```python
from build123d import *

# Parameters (mm, degrees)
SKETCH1_R           = 15
SKETCH1_R_2         = 40
BOSS_EXTRUDE4_DEPTH = 51


with BuildPart() as part:
    # Sketch1 → Boss-Extrude4 (new body)
    # profile 1 of 3: a face of its own
    with BuildSketch(Plane.XY):
        with BuildLine():
            ThreePointArc((-29.002885891, 59.651863383), (-46.6282273, 80.727545655), (-70.02485881, 66.324952937))
            Line((-70.02485881, 66.324952937), (-89.071294105, 6.023764702))
            ThreePointArc((-89.071294105, 6.023764702), (-66.95253237, 19.766460003), (-50, 0))
            ThreePointArc((-50, 0), (-66.95253237, -19.766460003), (-89.071294105, -6.023764702))
            Line((-89.071294105, -6.023764702), (-70.02485881, -66.324952937))
            ThreePointArc((-70.02485881, -66.324952937), (-46.6282273, -80.727545655), (-29.002885891, -59.651863383))
            ThreePointArc((-29.002885891, -59.651863383), (-22.168588856, -44.262528341), (-6.003756239, -39.546869801))
            ThreePointArc((-6.003756239, -39.546869801), (-40, 0), (-6.003756239, 39.546869801))
            ThreePointArc((-6.003756239, 39.546869801), (-22.168588856, 44.262528341), (-29.002885891, 59.651863383))
        make_face()
        with Locations((-50, -60)):
            Circle(SKETCH1_R, mode=Mode.SUBTRACT)
        with Locations((-50, 60)):
            Circle(SKETCH1_R, mode=Mode.SUBTRACT)
    # profile 2 of 3: a face of its own
    with BuildSketch(Plane.XY):
        with BuildLine():
            ThreePointArc((29.002885891, 59.651863383), (22.168588856, 44.262528341), (6.003756239, 39.546869801))
            ThreePointArc((6.003756239, 39.546869801), (30.332740146, 26.075369129), (40, 0))
            ThreePointArc((40, 0), (30.332740146, -26.075369129), (6.003756239, -39.546869801))
            ThreePointArc((6.003756239, -39.546869801), (22.168588856, -44.262528341), (29.002885891, -59.651863383))
            ThreePointArc((29.002885891, -59.651863383), (46.6282273, -80.727545655), (70.02485881, -66.324952937))
            Line((70.02485881, -66.324952937), (89.071294105, -6.023764702))
            ThreePointArc((89.071294105, -6.023764702), (50, 0), (89.071294105, 6.023764702))
            Line((89.071294105, 6.023764702), (70.02485881, 66.324952937))
            ThreePointArc((70.02485881, 66.324952937), (46.6282273, 80.727545655), (29.002885891, 59.651863383))
        make_face()
        with Locations((50, -60)):
            Circle(SKETCH1_R, mode=Mode.SUBTRACT)
        with Locations((50, 60)):
            Circle(SKETCH1_R, mode=Mode.SUBTRACT)
    # profile 3 of 3: a face of its own
    with BuildSketch(Plane.XY):
        Circle(SKETCH1_R_2)
        with BuildLine():
            ThreePointArc((26.090759323, 18.527608533), (16, 27.712812921), (3, 31.859064644))
            Line((3, 31.859064644), (3, 20.784609691))
            ThreePointArc((3, 20.784609691), (10.5, 18.186533479), (16.5, 12.990381057))
            Line((16.5, 12.990381057), (26.090759323, 18.527608533))
        make_face(mode=Mode.SUBTRACT)
        with BuildLine():
            Line((3, -20.784609691), (3, -31.859064644))
            ThreePointArc((3, -31.859064644), (16, -27.712812921), (26.090759323, -18.527608533))
            Line((26.090759323, -18.527608533), (16.5, -12.990381057))
            ThreePointArc((16.5, -12.990381057), (10.5, -18.186533479), (3, -20.784609691))
        make_face(mode=Mode.SUBTRACT)
        with BuildLine():
            Line((19.5, -7.794228634), (29.090759323, -13.331456111))
            ThreePointArc((29.090759323, -13.331456111), (32, 0), (29.090759323, 13.331456111))
            Line((29.090759323, 13.331456111), (19.5, 7.794228634))
            ThreePointArc((19.5, 7.794228634), (21, 0), (19.5, -7.794228634))
        make_face(mode=Mode.SUBTRACT)
        with BuildLine():
            Line((-3, 20.784609691), (-3, 31.859064644))
            ThreePointArc((-3, 31.859064644), (-16, 27.712812921), (-26.090759323, 18.527608533))
            Line((-26.090759323, 18.527608533), (-16.5, 12.990381057))
            ThreePointArc((-16.5, 12.990381057), (-10.5, 18.186533479), (-3, 20.784609691))
        make_face(mode=Mode.SUBTRACT)
        with BuildLine():
            Line((-19.5, 7.794228634), (-29.090759323, 13.331456111))
            ThreePointArc((-29.090759323, 13.331456111), (-32, 0), (-29.090759323, -13.331456111))
            Line((-29.090759323, -13.331456111), (-19.5, -7.794228634))
            ThreePointArc((-19.5, -7.794228634), (-21, 0), (-19.5, 7.794228634))
        make_face(mode=Mode.SUBTRACT)
        with BuildLine():
            Line((-16.5, -12.990381057), (-26.090759323, -18.527608533))
            ThreePointArc((-26.090759323, -18.527608533), (-16, -27.712812921), (-3, -31.859064644))
            Line((-3, -31.859064644), (-3, -20.784609691))
            ThreePointArc((-3, -20.784609691), (-10.5, -18.186533479), (-16.5, -12.990381057))
        make_face(mode=Mode.SUBTRACT)
    extrude(amount=BOSS_EXTRUDE4_DEPTH)


solid = part.part
```
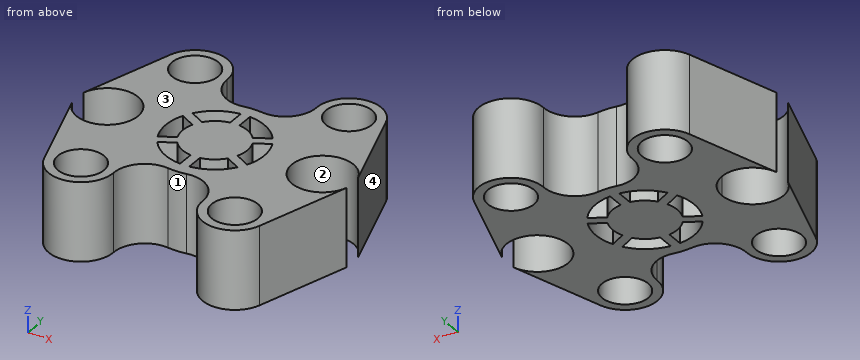
Work out the finished part from the listing and answer in its coordinate system (mm). Face numbers are marked on the shaded views. Coordinates: 2 decimals unless noted, no trailing zeros. Loops run counter-clockwise (first coordinate to the right, second up) from the corner with the lowest first, then second, coordinate; pieces in that order, holes last.
1) Section D-D (z = 4.5) is taken. Give the number of separate pieces and of enclosed holes in the cut face, plus the area to 3 significant figures.
Results:
separate pieces: 1
enclosed holes: 10
area: 13,500 mm2
2) Section C-C (x = -46.5) is taken. Give the vertices of the cut face in (y, z), plus the area to 3 significant figures.
Results:
outline: (-80.71, 0) - (-74.59, 0) - (-74.59, 51) - (-80.71, 51) - close; (-45.41, 0) - (45.41, 0) - (45.41, 51) - (-45.41, 51) - close; (74.59, 0) - (80.71, 0) - (80.71, 51) - (74.59, 51) - close
area: 5,260 mm2
3) Flat-ended cylindrical pins translate along their axes: pin 1 (1.5 mm diameter, centred on x = 60.5, z = 35.5, fed in from -Y); pin 2 (1.5 mm diameter, centred on y = 30, z = 42.5, fed in from -X); pin 3 (5 mm diameter, centred on y = -39, z = 20, fed in from +X). Find the tip coordinate at first contact, or state that the pin passes through.
Results:
pin 1: stops at y = -78.6
pin 2: stops at x = -81.74
pin 3: stops at x = 79.45
4) Consider probe 1 along Y at (x, z) = (49, 36); probe 2 along X at (y, z) = (58, 17.5); probe 3 along X at (y, z) = (16, 23.5). Determine where each line is inside the solid, lowest interval first.
Results:
probe 1: y = -80.98 to -74.97, -45.03 to 45.03, 74.97 to 80.98
probe 2: x = -72.65 to -64.87, -35.13 to -28.96, 28.96 to 35.13, 64.87 to 72.65
probe 3: x = -85.92 to -82, -58 to -21.71, -13.6 to 13.6, 21.71 to 58, 82 to 85.92
5) Section A-A (y = 2.5) is taken. Give the vertices of the cut face in (x, z).
Results:
outline: (-50.16, 0) - (-31.9, 0) - (-31.9, 51) - (-50.16, 51) - close; (-20.85, 0) - (20.85, 0) - (20.85, 51) - (-20.85, 51) - close; (31.9, 0) - (50.16, 0) - (50.16, 51) - (31.9, 51) - close
6) For a pull along Y with two mould halves and no side action, classify the marked faces 1, 2, 3 and 4 as +Y half, -Y half, draft (parallel to the pull), parting line (faces both ways), or undercut.
Results:
face 1: -Y half
face 2: undercut
face 3: draft
face 4: +Y half
7) Section B-B (x = 58.5) is taken. Give the vertices of the cut face in (y, z).
Results:
outline: (-79.2, 0) - (-72.36, 0) - (-72.36, 51) - (-79.2, 51) - close; (-47.64, 0) - (-16.36, 0) - (-16.36, 51) - (-47.64, 51) - close; (16.36, 0) - (47.64, 0) - (47.64, 51) - (16.36, 51) - close; (72.36, 0) - (79.2, 0) - (79.2, 51) - (72.36, 51) - close
